Work out the finished part from the listing and answer in its coordinate system (mm). A direction names the side the tool comes from. Give positions to 0.01 mm unless a question says otherwise; leave off trailing zeros. Loops run counter-clockwise (first coordinate to the right, second up) from the corner with the lowest first, then second, coordinate; pieces in that order, holes last. Notation, with made-up numbers: (17.25, -19) - (65.25, -19) arc R21 ccw to (65.25, 2) - close; hole circle Ø3 at (76, -4). An arc over 180 degrees is marked (long way). One line per question, with ' | ' between items. Start each with the question number.
1. Find the intervals of material crossed by line 1 (X direction, y = 68.5, z = -4.5); line 2 (Y direction, x = 20.5, z = -12); line 3 (X direction, y = 68.5, z = 20), in increasing order.
2. Section B-B (z = 0) is taken. Determine the outline of the cut face in (x, y).
3. Which of the six approach directions +Z, -Z, +X, -X, +Y, -Y give full straight-line access (tool end or side, diameter ignored) to faces 4 (the face through (0, 12, 0)), 5 (the face through (-45.644, 43.384, 0.19)), 6 (the face through (0, 54, 20.4))?
4. Section C-C (y = 45) is taken. Determine the outline of the cut face in (x, z) (3 decimals).
5. For a pull along Z with two mould halves and no side action, classify faces 1 (the face through (0, 6, 10.424)), 2 (the face through (-1, 88, 22)), 3 (the face through (-10.902, 43.384, 49.096)) as released by +Z, released by -Z, zero draft, split by the parting line, or undercut.
6. Section D-D (x = 0) is taken. Determine the outline of the cut face in (y, z), plus the area to 3 significant figures.
7. Section A-A (x = -38) is taken. Determine the outline of the cut face in (y, z).
8. Each of these flat-tipped pins is pushed along its axis until it touches: pin 1 (3.5 mm diameter, centred on y = 7.5, z = -2, fed in from +X); pin 2 (13 mm diameter, centred on x = -4.5, y = 3.5, fed in from -Z); pin 3 (6 mm diameter, centred on y = 33.5, z = 29, fed in from -X). Where does it stop, or does it pass through?
from build123d import *

# Parameters (mm, degrees)
SKETCH1_R           = 50.292
SKETCH1_R_2         = 3.475
BOSS_EXTRUDE1_DEPTH = 88
SKETCH2_W           = 60.822109288
SKETCH2_H           = 40.800022246
CUT_EXTRUDE1_DEPTH  = 68.04
SKETCH3_W           = 49.01906667
SKETCH3_H           = 20.847628368
CUT_EXTRUDE2_DEPTH  = 12


with BuildPart() as part:
    # Sketch1 → Boss-Extrude1 (new body)
    with BuildSketch(Plane(origin=(0, 0, 0), x_dir=(1, 0, 0), z_dir=(0, 1, 0))):
        Circle(SKETCH1_R)
        with Locations((42.886820356, 1.924977859)):
            Circle(SKETCH1_R_2, mode=Mode.SUBTRACT)
        with Locations((-42.886820356, 1.924977859)):
            Circle(SKETCH1_R_2, mode=Mode.SUBTRACT)
        with Locations((-37.000474826, -12.718618748)):
            Circle(SKETCH1_R_2, mode=Mode.SUBTRACT)
        with Locations((-23.129730363, 31.556520301)):
            Circle(SKETCH1_R_2, mode=Mode.SUBTRACT)
        with Locations((37.000474826, -12.718618748)):
            Circle(SKETCH1_R_2, mode=Mode.SUBTRACT)
        with Locations((23.129730363, 31.556520301)):
            Circle(SKETCH1_R_2, mode=Mode.SUBTRACT)
    extrude(amount=BOSS_EXTRUDE1_DEPTH)

    # Sketch2 → Cut-Extrude1 (cut)
    with BuildSketch(Plane(origin=(0, 88, 0), x_dir=(1, 0, 0), z_dir=(0, 1, 0))):
        Rectangle(SKETCH2_W, SKETCH2_H)
    extrude(amount=-CUT_EXTRUDE1_DEPTH, mode=Mode.SUBTRACT)

    # Sketch3 → Cut-Extrude2 (cut)
    with BuildSketch(Plane(origin=(0, 0, 0), x_dir=(-1, 0, 0), z_dir=(0, -1, 0))):
        Rectangle(SKETCH3_W, SKETCH3_H)
    extrude(amount=-CUT_EXTRUDE2_DEPTH, mode=Mode.SUBTRACT)


solid = part.part
Conclusion:
1) line 1: -50.09 to -45.22, -40.55 to -30.41, 30.41 to 40.55, 45.22 to 50.09 | line 2: 0 to 19.96 | line 3: -46.14 to -30.41, 30.41 to 46.14
2) outline: (-50.29, 0) - (-45.78, 0) - (-45.78, 88) - (-50.29, 88) - close; (-39.99, 0) - (-24.51, 0) - (-24.51, 12) - (24.51, 12) - (24.51, 0) - (39.99, 0) - (39.99, 88) - (30.41, 88) - (30.41, 19.96) - (-30.41, 19.96) - (-30.41, 88) - (-39.99, 88) - close; (45.78, 0) - (50.29, 0) - (50.29, 88) - (45.78, 88) - close
3) face 4: -Y | face 5: +Y, -Y | face 6: +Y
4) outline: circle Ø100.584 at (0, 0); hole circle Ø6.95 at (-42.887, -1.925); hole circle Ø6.95 at (-37, 12.719); hole (-30.411, -20.4) - (30.411, -20.4) - (30.411, 20.4) - (-30.411, 20.4) - close; hole circle Ø6.95 at (-23.13, -31.557); hole circle Ø6.95 at (23.13, -31.557); hole circle Ø6.95 at (37, 12.719); hole circle Ø6.95 at (42.887, -1.925)
5) face 1: undercut | face 2: zero draft | face 3: split by the parting line
6) outline: (0, -50.29) - (88, -50.29) - (88, -20.4) - (19.96, -20.4) - (19.96, 20.4) - (88, 20.4) - (88, 50.29) - (0, 50.29) - (0, 10.42) - (12, 10.42) - (12, -10.42) - (0, -10.42) - close | area: 5,830 mm²
7) outline: (0, -32.94) - (88, -32.94) - (88, 9.39) - (0, 9.39) - close; (0, 16.05) - (88, 16.05) - (88, 32.94) - (0, 32.94) - close
8) pin 1: x = 50.29 | pin 2: z = -50.29 | pin 3: x = -43.05
